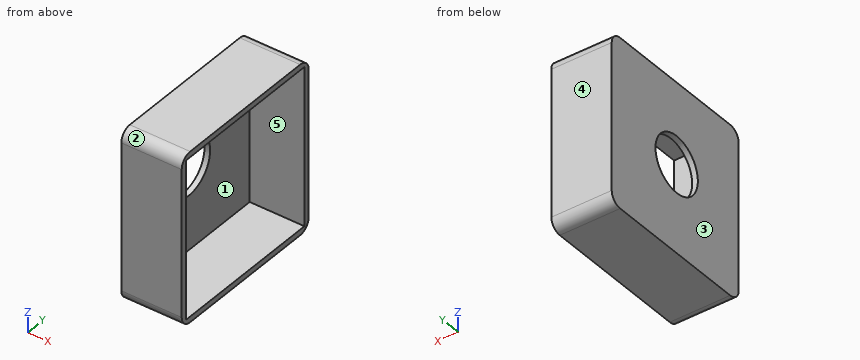
```python
from build123d import *

# Parameters (mm, degrees)
F1_DEPTH = 27.14701
F2_T     = -2.54
F3_R     = 5.08
F4_R     = 12.7
F5_DEPTH = 51.567206


with BuildPart() as f1:
    # F0 (on Right) → F1 (new body)
    with BuildSketch(Plane.YZ):
        Polygon((-28.252147, 57.261179), (-66.352147, 57.261179), (-66.352147, -18.938821), (9.847853, -18.938821), (9.847853, 57.261179), align=None)
    extrude(amount=F1_DEPTH)

    # F2
    f2_openings = [f1.faces().sort_by_distance(p)[0] for p in [
        (27.14701, -28.252147, 19.161179),
    ]]
    offset(amount=F2_T, openings=f2_openings)

    # F3
    f3_edges = [f1.edges().sort_by_distance(p)[0] for p in [
        (13.573505, 9.847853, -18.938821),
        (13.573505, 9.847853, 57.261179),
        (13.573505, -66.352147, -18.938821),
        (13.573505, -66.352147, 57.261179),
    ]]
    fillet(f3_edges, radius=F3_R)

    # F4 (on face) → F5 (cut)
    with BuildSketch(Plane.YZ.offset(2.54)):
        with Locations((-29.138448, 20.637747)):
            Circle(F4_R)
    extrude(amount=-F5_DEPTH, mode=Mode.SUBTRACT)


solid = f1.part
```
Check sheet for the modelled part. Datum: model origin and axes. Units: mm. Face numbers are marked on the shaded views. A direction names the side the tool comes from. Round coordinates to 2 decimals unless told otherwise and drop trailing zeros. Order: outer loops, then holes, each group sorted by start corner. A loop starts at its lowest first (then second) coordinate and runs counter-clockwise, first axis right, second up.
1) Section check A-A (x = 15). Record the boundary of the cut face in (y, z).
2) Mould release check, pull along Y, two halves, no side actions. Record for the marked faces 1, 2 and 3: +Y half, -Y half, draft (parallel to the pull), parting line (faces both ways), or undercut.
3) Section check B-B (y = -9). Record the boundary of the cut face in (x, z).
4) Section check C-C (z = 27.5). Record the boundary of the cut face in (x, y), and give its area (3 significant figures).
5) Section check D-D (z = 6). Record the boundary of the cut face in (x, y).
6) Tool access check on the marked faces 4 and 5. Record the directions out of +Z, -Z, +X, -X, +Y, -Y that give a thin tool (end or side, any length) a straight path to the whole face; none if there is none.
7) Scan lines: line 1 (Y direction, x = 12, z = 33.5); line 2 (Z direction, x = 9.75, y = -44); line 3 (X direction, y = 5, z = -2). Record each from-to range of solid material in increasing order.
8) Go/stop test with a flat-tipped pin: pin 1 Ø5 at (y, z) = (-13.5, 5) entering from +X. Record where the tip stops, or that it passes through.
Result:
1. outline: (-66.35, -13.86) arc R5.08 ccw to (-61.27, -18.94) - (4.77, -18.94) arc R5.08 ccw to (9.85, -13.86) - (9.85, 52.18) arc R5.08 ccw to (4.77, 57.26) - (-61.27, 57.26) arc R5.08 ccw to (-66.35, 52.18) - close; hole (-63.81, -16.4) - (7.31, -16.4) - (7.31, 54.72) - (-63.81, 54.72) - close
2. face 1: undercut
2. face 2: -Y half
2. face 3: draft
3. outline: (0, -18.94) - (27.15, -18.94) - (27.15, -16.4) - (2.54, -16.4) - (2.54, 54.72) - (27.15, 54.72) - (27.15, 57.26) - (0, 57.26) - close
4. outline: (0, -66.35) - (27.15, -66.35) - (27.15, -63.81) - (2.54, -63.81) - (2.54, -39.82) - (0, -39.82) - close; (0, -18.45) - (2.54, -18.45) - (2.54, 7.31) - (27.15, 7.31) - (27.15, 9.85) - (0, 9.85) - close
4. area: 264 mm2
5. outline: (0, -66.35) - (27.15, -66.35) - (27.15, -63.81) - (2.54, -63.81) - (2.54, 7.31) - (27.15, 7.31) - (27.15, 9.85) - (0, 9.85) - close
6. face 4: +Z, -Z, +X, -X, +Y
6. face 5: +X
7. line 1: y = -66.35 to -63.81, 7.31 to 9.85
7. line 2: z = -18.94 to -16.4, 54.72 to 57.26
7. line 3: x = 0 to 2.54
8. pin 1: stops at x = 2.54
